For this review, take the finished solid that the model builds, in its own axes (mm). A direction names the side the tool comes from. Give positions to 0.01 mm unless a question says otherwise; leave off trailing zeros. Loops run counter-clockwise (first coordinate to the right, second up) from the corner with the lowest first, then second, coordinate; pieces in that order, holes last. Notation, with made-up numbers: (18.5, -27) - (69.5, -27) arc R13 cw to (69.5, -14) - close; hole circle Ø10 at (17, 17.5). An arc over 180 degrees is marked (long way). Put each result on its own line as item: value.
from build123d import *

# Parameters (mm, degrees)
F0_R     = 13.97
F1_DEPTH = 3.175
F2_R     = 1.27
F3_R     = 7.62
F3_R_2   = 5.08
F4_DEPTH = 0.3175
F5_R     = 2.5019
F6_DEPTH = 4
F7_R     = 1.016
F8_DEPTH = 0.3175


with BuildPart() as f1:
    # F0 (on Front) → F1 (new body, symmetric)
    with BuildSketch(Plane.XZ):
        Circle(F0_R)
    extrude(amount=F1_DEPTH, both=True)

    # F2
    f2_edges = [f1.edges().sort_by_distance(p)[0] for p in [
        (-13.97, -3.175, 0),
        (-13.97, 3.175, 0),
    ]]
    fillet(f2_edges, radius=F2_R)

    # F3 (on face) → F4 (cut)
    with BuildSketch(Plane.XZ.offset(3.175)):
        Circle(F3_R)
        Circle(F3_R_2, mode=Mode.SUBTRACT)
    extrude(amount=-F4_DEPTH, mode=Mode.SUBTRACT)

    # F5 (on face) → F6 (join)
    with BuildSketch(Plane(origin=(0, 3.175, 0), x_dir=(-1, 0, 0), z_dir=(0, 1, 0))):
        Circle(F5_R)
    extrude(amount=F6_DEPTH)

    # F7 (on face) → F8 (cut)
    with BuildSketch(Plane.XZ.offset(2.8575)):
        with Locations((0, 6.35)):
            Circle(F7_R)
        with Locations((0, -6.35)):
            Circle(F7_R)
        with Locations((-6.35, 0)):
            Circle(F7_R)
        with Locations((6.35, 0)):
            Circle(F7_R)
        with BuildLine():
            ThreePointArc((-5.208549, 5.208549), (-5.208549, 3.771708), (-3.771708, 3.771708))
            Line((-3.771708, 3.771708), (-5.208549, 5.208549))
        make_face()
        with BuildLine():
            Line((-5.208549, 5.208549), (-3.771708, 3.771708))
            ThreePointArc((-3.771708, 3.771708), (-3.551466, 4.101322), (-3.474128, 4.490128))
            ThreePointArc((-3.474128, 4.490128), (-4.101322, 5.42879), (-5.208549, 5.208549))
        make_face()
        with BuildLine():
            ThreePointArc((5.350396, -4.490128), (4.819338, -3.695344), (3.881827, -3.881827))
            Line((3.881827, -3.881827), (5.09843, -5.09843))
            ThreePointArc((5.09843, -5.09843), (5.284912, -4.819338), (5.350396, -4.490128))
        make_face()
        with BuildLine():
            Line((5.09843, -5.09843), (3.881827, -3.881827))
            ThreePointArc((3.881827, -3.881827), (3.881827, -5.09843), (5.09843, -5.09843))
        make_face()
        with BuildLine():
            ThreePointArc((-3.567395, -4.490128), (-3.637633, -4.137013), (-3.837657, -3.837657))
            Line((-3.837657, -3.837657), (-5.142599, -5.142599))
            ThreePointArc((-5.142599, -5.142599), (-4.137013, -5.342623), (-3.567395, -4.490128))
        make_face()
        with BuildLine():
            Line((-5.142599, -5.142599), (-3.837657, -3.837657))
            ThreePointArc((-3.837657, -3.837657), (-5.142599, -3.837657), (-5.142599, -5.142599))
        make_face()
        with BuildLine():
            ThreePointArc((5.208549, 5.208549), (3.771708, 5.208549), (3.771708, 3.771708))
            Line((3.771708, 3.771708), (5.208549, 5.208549))
        make_face()
        with BuildLine():
            Line((5.208549, 5.208549), (3.771708, 3.771708))
            ThreePointArc((3.771708, 3.771708), (4.878934, 3.551466), (5.506128, 4.490128))
            ThreePointArc((5.506128, 4.490128), (5.42879, 4.878934), (5.208549, 5.208549))
        make_face()
    extrude(amount=-F8_DEPTH, mode=Mode.SUBTRACT)


solid = f1.part
1) For faces 5 (the face through (2, 5.1, -1.5)), 6 (the face through (5, -2.858, -2)), 7 (the face through (0, -3.175, 0)), list the 3-axis set-ups (+Z, -Z, +X, -X, +Y, -Y) from which the entire face can be reached by the end or side of a thin tool; tool diameter is ignored.
Geometry check:
face 5: +Y
face 6: -Y
face 7: +Z, -Z, +X, -X, -Y
2) Wall thickness on line 1 (Z direction, x = 0, y = -2.7); line 2 (Y direction, x = 1.75, z = -8) (3 decimals); line 3 (Y direction, x = 7.5, z = 0) (1 decimal): over which ranges is each line inside the solid? List them lowest first.
Geometry check:
line 1: z = -13.69 to -7.37, -5.33 to 5.33, 7.37 to 13.69
line 2: y = -3.175 to 3.175
line 3: y = -2.9 to 3.2
3) Insertion check: pin 1 Ø1.8 at (x, z) = (6.35, 0) entering from -Y; pin 2 Ø2 at (x, z) = (6.5, -0.5) entering from -Y; pin 3 Ø2.5 at (x, z) = (0, 6.35) entering from +Y (3 decimals); pin 4 Ø3.5 at (x, z) = (0, -6.35) entering from -Y (3 decimals). Each pin has a flat end and moves straight along its axis. Give the tip position at first contact, or say it passes through.
Geometry check:
pin 1: stops at y = -2.54
pin 2: stops at y = -2.86
pin 3: stops at y = 3.175
pin 4: stops at y = -3.175
4) Draft analysis for pull direction Z (two halves, no side actions). For faces 1 (the face through (4, -2.54, 5)), 2 (the face through (-0.661, -3.018, 5.037)), 3 (the face through (3, 3.175, 0)), 4 (the face through (-1.82, -0.03, 13.85)), state which applies: pulls with the +Z half, pulls with the -Z half, needs draft (parallel to the pull), parting line crosses it, or undercut.
Geometry check:
face 1: undercut
face 2: undercut
face 3: needs draft
face 4: parting line crosses it
5) Take a section at C-C on y = 4.25. State the section outline as (x, z) points, and give its area (3 significant figures).
Geometry check:
outline: circle Ø5 at (0, 0)
area: 19.7 mm²
